Part print with two shaded views. Sizes in mm from the minimum x, y, z corner. A direction names the side the tool comes from. Give positions to 0.01 mm unless a question says otherwise; leave off trailing zeros. Write each loop counter-clockwise with the first axis right and the second up, starting at its lowest first coordinate (ties: lowest second). Pieces come first, ordered by that corner, then holes. Notation, with made-up numbers: M -25,-16.5 L -11,-16.5 A18 cw -11,-5.5 Z; hole C -24,38.25 d8. An arc over 180 degrees is marked long. One line per item, written item: value. Start each with the question number.
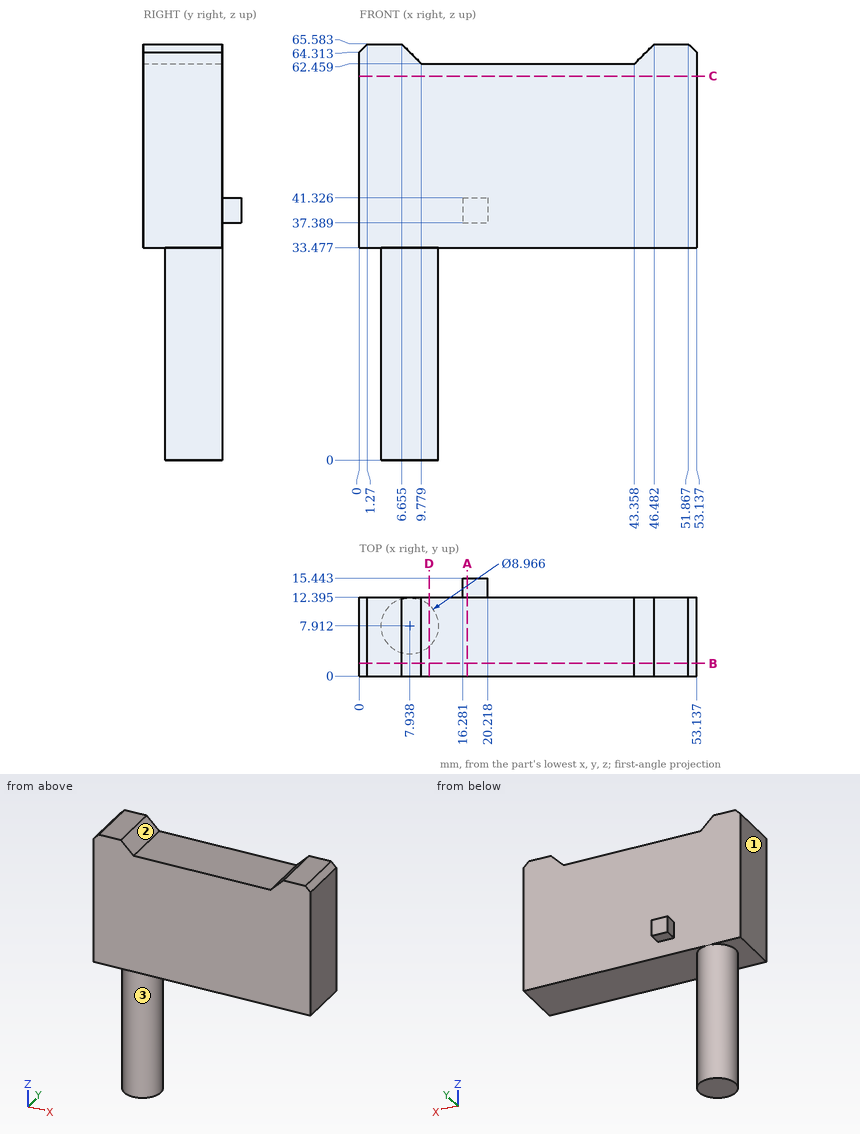
1) Band-saw the part on B-B (y = 2). List the corners of the cut face in (x, z) (1 decimal).
2) Band-saw the part on A-A (x = 17). List the corners of the cut face in (y, z) (1 decimal).
3) Drop flat-ended pins along their axis: P1, Ø2, axis at x = 27, y = 6.5, coming from the +Z side; P2, Ø8, axis at y = 11.5, z = 10, coming from the -X side; P3, Ø1, axis at x = 40, z = 56.5, coming from the +Y side (1 decimal). Give the stop position or say it passes through.
4) Band-saw the part on D-D (x = 11). List the corners of the cut face in (y, z) (1 decimal).
5) Band-saw the part on C-C (z = 60.5). List the corners of the cut face in (x, y) (1 decimal), then the cut area to 3 significant figures.
6) Probe line 1 along Z through (x, y) = (23, 2.5); line 2 along X through (y, z) = (13, 38.5); line 3 along Z through (x, y) = (49.5, 11). List the from-to ranges inside material, lowest first. Write a range as from..to.
7) Tool access for the marked faces 1, 2 and 3: list every direction of +Z, -Z, +X, -X, +Y, -Y with a clear straight run to the whole face (end or side of a thin tool).
Model answer:
1. outline: M 0,33.5 L 53.1,33.5 L 53.1,64.3 L 51.9,65.6 L 46.5,65.6 L 43.4,62.5 L 9.8,62.5 L 6.7,65.6 L 1.3,65.6 L 0,64.3 Z
2. outline: M 0,33.5 L 12.4,33.5 L 12.4,37.4 L 15.4,37.4 L 15.4,41.3 L 12.4,41.3 L 12.4,62.5 L 0,62.5 Z
3. P1: stops at z = 62.46
3. P2: stops at x = 3.45
3. P3: stops at y = 12.4
4. outline: M 0,33.5 L 4.6,33.5 L 4.6,0 L 11.2,0 L 11.2,33.5 L 12.4,33.5 L 12.4,62.5 L 0,62.5 Z
5. outline: M 0,0 L 53.1,0 L 53.1,12.4 L 0,12.4 Z
5. area: 659 mm²
6. line 1: z = 33.48..62.46
6. line 2: x = 16.28..20.22
6. line 3: z = 33.48..65.58
7. face 1: +Z, -Z, -X, +Y, -Y
7. face 2: +Z, +Y, -Y
7. face 3: -Z
